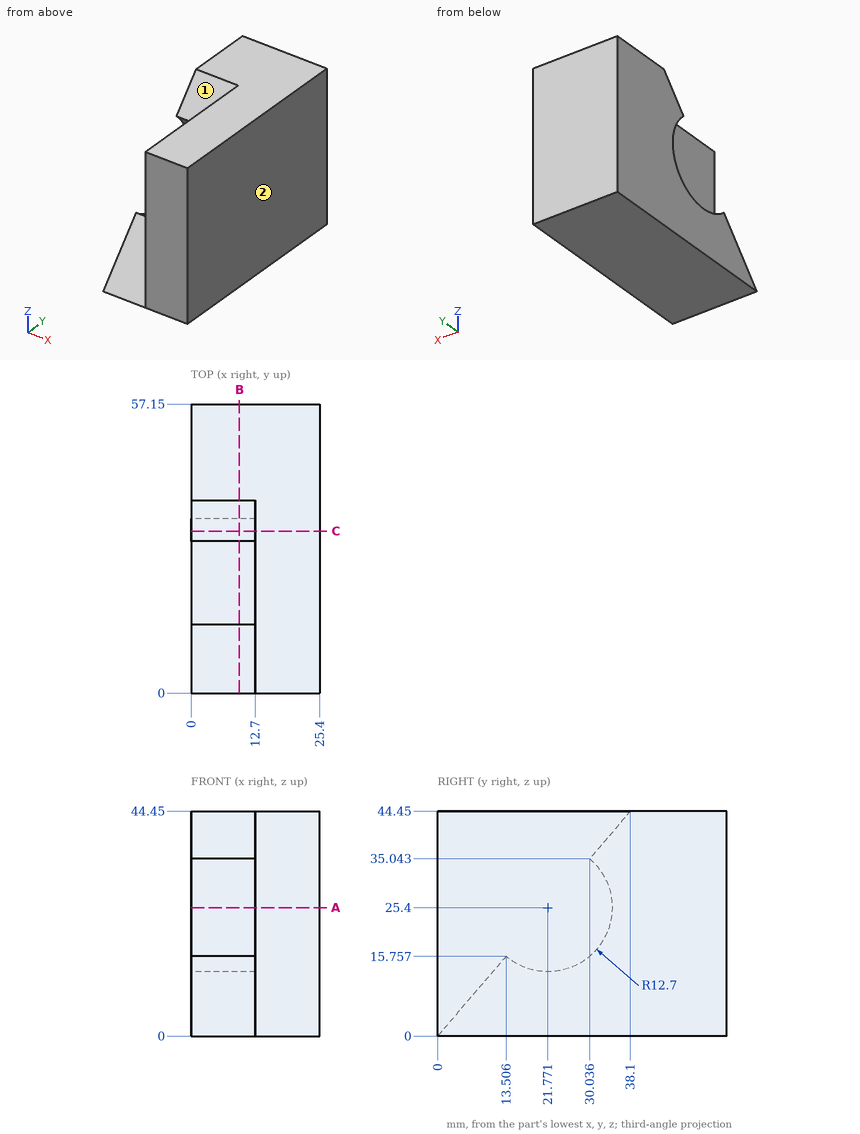
The figure shows three views and two pictorial views of one solid part (mm, origin at its lowest corner). Answer the questions. A direction names the side the tool comes from. Give positions to 0.01 mm unless a question says otherwise; leave off trailing zeros. Loops run counter-clockwise (first coordinate to the right, second up) from the corner with the lowest first, then second, coordinate; pieces in that order, holes last. Notation, with made-up numbers: (73, -13.5) - (93, -13.5) arc R18 ccw to (93, 12.5) - close; hole circle Ø7 at (83.25, 23.5). An arc over 180 degrees is marked (long way). Answer in a Markdown table with one row per item.
(1) Consider L1, parallel to X at y = 18.5, z = 27.5; L2, parallel to Z at x = 8.25, y = 22; L3, parallel to Y at x = 4, z = 25.5. Determine where each line is inside the solid, lowest interval first. Write a range as [from, to].
Results list:
| item | result |
|---|---|
| L1 | x = [12.7, 25.4] |
| L2 | z = [0, 12.7] |
| L3 | y = [34.47, 57.15] |
(2) A tool of negligible diameter and unlimited length cuts with its end or side. For the marked faces 1 and 2, from which of +Z, -Z, +X, -X, +Y, -Y can it reach the whole face along a straight path? Write none if from no direction.
Results list:
| item | result |
|---|---|
| face 1 | +Z, -X, -Y |
| face 2 | +Z, -Z, +X, +Y, -Y |
(3) Section B-B (x = 9.5) is taken. Give the vertices of the cut face in (y, z), and give its area (3 significant figures).
Results list:
| item | result |
|---|---|
| outline | (0, 0) - (57.15, 0) - (57.15, 44.45) - (38.1, 44.45) - (30.04, 35.04) arc R12.7 cw to (13.51, 15.76) - close |
| area | 1,440 mm² |
(4) Section A-A (z = 25.4) is taken. Give the vertices of the cut face in (x, y).
Results list:
| item | result |
|---|---|
| outline | (0, 34.47) - (12.7, 34.47) - (12.7, 0) - (25.4, 0) - (25.4, 57.15) - (0, 57.15) - close |
(5) Section C-C (y = 32) is taken. Give the vertices of the cut face in (x, z).
Results list:
| item | result |
|---|---|
| outline | (0, 0) - (25.4, 0) - (25.4, 44.45) - (12.7, 44.45) - (12.7, 37.33) - (0, 37.33) - (0, 32.93) - (12.7, 32.93) - (12.7, 17.87) - (0, 17.87) - close |
(6) A flat-ended cylindrical pin translates along its axis: pin 1 Ø10 at (y, z) = (9.5, 19) entering from -X. Find the tip coordinate at first contact, or state that the pin passes through.
Results list:
| item | result |
|---|---|
| pin 1 | stops at x = 12.7 |
